from build123d import *

# Parameters (mm, degrees)
F0_R     = 9.525
F2_R     = 22.225
F6_R     = 19.05
F7_DEPTH = 6.35
F5_R     = 7.62
F4_R     = 20.32
F9_R     = 2.54


with BuildPart() as f3:
    # F0 (on Top) → F3 section 0
    with BuildSketch(Plane.XY):
        Circle(F0_R)
    # F2 (on offset) → F3 section 1
    with BuildSketch(Plane.XY.offset(124.46)):
        Circle(F2_R)
    loft()

    # F6 (on Top) → F7 (join)
    with BuildSketch(Plane.XY):
        Circle(F6_R)
    extrude(amount=F7_DEPTH)

    # F5 (on face) → F8 section 0
    with BuildSketch(Plane(origin=(0, 0, 0), x_dir=(1, 0, 0), z_dir=(0, 0, -1))):
        Circle(F5_R)
    # F4 (on face) → F8 section 1
    with BuildSketch(Plane.XY.offset(124.46)):
        Circle(F4_R)
    loft(mode=Mode.SUBTRACT)

    # F9
    f9_edges = [f3.edges().sort_by_distance(p)[0] for p in [
        (-19.05, 0, 6.35),
        (-19.05, 0, 0),
    ]]
    fillet(f9_edges, radius=F9_R)


solid = f3.part
Verification items for the finished model (mm, model axes). A direction names the side the tool comes from. Coordinates: 2 decimals unless noted, no trailing zeros. Loops run counter-clockwise (first coordinate to the right, second up) from the corner with the lowest first, then second, coordinate; pieces in that order, holes last. Notation, with made-up numbers: (46, 77) -> (57, 77) arc R26 ccw to (57, 103) -> close; hole circle Ø6 at (-22, 60.5). An arc over 180 degrees is marked (long way). Answer as a JSON object with one key per item and string values. Group by question number.
Item 1: Sectioned sample at B-B on z = 84. Record the boundary of the cut face in (x, y), plus the area to 3 significant figures.
Item 2: Sectioned sample at C-C on z = 62. Record the boundary of the cut face in (x, y), plus the area to 3 significant figures.
Item 3: Mould release check, pull along X, two halves, no side actions. Record for faces 4 (the flat face through (3.4, -7.1, 0)), 5 (the conical face through (-12.92, -9.91, 66.23)), 6 (the conical face through (13.41, -4.22, 63.1)): +X half, -X half, draft (parallel to the pull), parting line (faces both ways), or undercut.
Item 4: Depth check by flat-ended pin: pin 1 (8 mm diameter, centred on y = 14, z = 98, fed in from -X); pin 2 (3 mm diameter, centred on x = 11.5, y = 14.5, fed in from -Z); pin 3 (2 mm diameter, centred on y = -8, z = 42, fed in from -X). Enter the tip coordinate at first touch or a pass-through.
Item 5: Scan lines: probe 1 along Y at (x, z) = (-5, 28); probe 2 along Y at (x, z) = (4, 52); probe 3 along X at (y, z) = (-13, 109.5). Record each from-to range of solid material in increasing order.
Item 6: Sectioned sample at A-A on x = 0. Record the boundary of the cut face in (y, z) (3 decimals).
Item 7: Tool access check on faces 1 (the flat face through (10, -18, 124.46)), 2 (the flat face through (-8, -7, 6.35)), 3 (the cylindrical face through (-15.12, -11.59, 3.17)). Record the directions out of +Z, -Z, +X, -X, +Y, -Y that give a thin tool (end or side, any length) a straight path to the whole face; none if there is none.
Evaluation:
{
 "1": {"outline": "circle Ø36.19 at (0, 0); hole circle Ø32.38 at (0, 0)", "area": "205 mm²"},
 "2": {"outline": "circle Ø31.7 at (0, 0); hole circle Ø27.89 at (0, 0)", "area": "178 mm²"},
 "3": {"face 4": "draft", "face 5": "parting line", "face 6": "undercut"},
 "4": {"pin 1": "stops at x = -16.82", "pin 2": "stops at z = 0.05", "pin 3": "stops at x = -11.92"},
 "5": {"probe 1": "y = -11.33 to -9.21, 9.21 to 11.33", "probe 2": "y = -14.28 to -12.29, 12.29 to 14.28", "probe 3": "x = -16.11 to -13.57, 13.57 to 16.11"},
 "6": {"outline": "(-22.225, 124.46) -> (-10.173, 6.35) -> (-16.51, 6.35) arc R2.54 ccw to (-19.05, 3.81) -> (-19.05, 2.54) arc R2.54 ccw to (-16.51, 0) -> (-7.62, 0) -> (-20.32, 124.46) -> close; (7.62, 0) -> (16.51, 0) arc R2.54 ccw to (19.05, 2.54) -> (19.05, 3.81) arc R2.54 ccw to (16.51, 6.35) -> (10.173, 6.35) -> (22.225, 124.46) -> (20.32, 124.46) -> close"},
 "7": {"face 1": "+Z, +X, -X, +Y, -Y", "face 2": "none", "face 3": "-Z"}
}
